Autodesk Inventor part; units mm, degrees
ref_plane "YZ Plane" through (0, 0, 0) normal (1, 0, 0) x (0, 1, 0)
ref_plane "XZ Plane" through (0, 0, 0) normal (0, 1, 0) x (-1, 0, 0)
ref_plane "XY Plane" through (0, 0, 0) normal (0, 0, 1) x (1, 0, 0)
sketch "Sketch1" plane through (0, 0, 0) normal (1, 0, 0) x (0, 1, 0)
  line L0 (25.4, 25.4) -> (25.4, -114.1235)
  arc A0 (-12.6706, -115.1818) -> (25.4, -114.1235) centre (6.35, -114.1235) ccw
  line L1 (-20.4928, 25.4) -> (-12.6706, -115.1818)
  circle A1 centre (0, 0) radius 11.1125
  circle A2 centre (6.35, -114.1235) radius 11.1125
  line L2 (6.35, -114.1235) -> (0, 0) construction
  line L3 (25.4, 25.4) -> (-20.4928, 25.4)
  circle A3 centre (-3.175, -37.9675) radius 11.1125
  circle A4 centre (6.35, -114.1235) radius 9.525 construction
  circle A5 centre (6.35, -114.1235) radius 15.875 construction
  line L4 (15.875, -15.875) -> (15.875, 15.875) construction
  line L5 (15.875, 15.875) -> (-15.875, 15.875) construction
  circle A6 centre (15.875, 15.875) radius 1.5875
  circle A7 centre (-15.875, 15.875) radius 1.5875
  circle A8 centre (15.875, -15.875) radius 1.5875
  point P0 (6.8794, -133.1661)
  dimension "d1" = 114.3
  dimension "d2" = 6.35
  dimension "d3" = 22.225
  dimension "d9" = 25.4
  dimension "d10" = 25.4
  dimension "d11" = 19.05
  dimension "d12" = 38.1
  dimension "d13" = 3.175
  dimension "d14" = 19.05
  dimension "d15" = 6.35
  dimension "d25" = 3.175
  dimension "d26" = 9.525
  dimension "d27" = 9.525
  dimension "d28" = 31.75
extrude "Extrusion1" add sketch "Sketch1" along normal blind 3.175
properties part number "Hopper pully plate"
Part model, mm, in its own coordinate system. Coordinates: 2 decimals unless noted, no trailing zeros. Order: outer loops, then holes, each group sorted by start corner. A loop starts at its lowest first (then second) coordinate and runs counter-clockwise, first axis right, second up. Notation, with made-up numbers: (-34, 53.25) - (22, 53.25) arc R19 cw to (22, 85.25) - close; hole circle Ø6 at (-10, 45.5). An arc over 180 degrees is marked (long way). Return JSON: item names as keys, results as strings. Group by question number.
Item 1: Drill centre lines: probe 1 along Z at (x, y) = (2.25, 0); probe 2 along Z at (x, y) = (0.65, 4); probe 3 along Z at (x, y) = (3, 9). Where is each one in solid material? Low to high. Write a range as from..to.
Item 2: Pull direction Z, two halves, no side cores. Call faces 1 (the face through (1.565, 15.531, 17.425)), 2 (the face through (2, 25.4, -43)), 3 (the face through (2, 3, 25.4)): pulls with the +Z half, pulls with the -Z half, needs draft (parallel to the pull), parting line crosses it, or undercut.
Item 3: Cut at C-C (x = 0.65). State how many separate pieces and enclosed holes the cut face has, plus the area to 3 significant figures.
Item 4: Cut at A-A (z = -105). List the corners of the cut face in (x, y) (3 decimals), plus the area to 3 significant figures.
Item 5: Cut at B-B (y = 0). List the corners of the cut face in (x, z) (1 decimal), plus the area to 3 significant figures.
Item 6: Cut at D-D (z = 0). List the corners of the cut face in (x, y) (1 decimal).
Check values:
{
 "1": {"probe 1": "z = -132.08..-123.24, -105..-48.62, -27.32..-11.11, 11.11..25.4", "probe 2": "z = -133.03..-124.98, -103.26..-46.45, -29.48..-10.37, 10.37..25.4", "probe 3": "z = -132.99..-124.92, -103.33..-6.52, 6.52..25.4"},
 "2": {"face 1": "undercut", "face 2": "needs draft", "face 3": "pulls with the +Z half"},
 "3": {"separate pieces": "1", "enclosed holes": "6", "area": "5,240 mm2"},
 "4": {"outline": "(0, -13.237) - (3.175, -13.237) - (3.175, 0.006) - (0, 0.006) - close; (0, 12.694) - (3.175, 12.694) - (3.175, 25.4) - (0, 25.4) - close", "area": "82.4 mm2"},
 "5": {"outline": "(0, -132.1) - (3.2, -132.1) - (3.2, -123.2) - (0, -123.2) - close; (0, -105) - (3.2, -105) - (3.2, -48.6) - (0, -48.6) - close; (0, -27.3) - (3.2, -27.3) - (3.2, -11.1) - (0, -11.1) - close; (0, 11.1) - (3.2, 11.1) - (3.2, 25.4) - (0, 25.4) - close", "area": "304 mm2"},
 "6": {"outline": "(0, -19.1) - (3.2, -19.1) - (3.2, -11.1) - (0, -11.1) - close; (0, 11.1) - (3.2, 11.1) - (3.2, 25.4) - (0, 25.4) - close"}
}
